```python
from build123d import *

# Parameters (mm, degrees)
SKETCH_W        = 500
SKETCH_H        = 800
PAD_DEPTH       = 850
SKETCH001_W     = 372.739898
SKETCH001_H     = 785.491455
SKETCH001_W_2   = 349.575272
SKETCH001_H_2   = 785.491421
POCKET_DEPTH    = 5
SKETCH002_W     = 52.646911
SKETCH002_H     = 789.7032
PAD001_DEPTH    = 150
SKETCH003_W     = 357.712269
SKETCH003_H     = 667.311138
POCKET001_DEPTH = 5
SKETCH004_W     = 152.212128
SKETCH004_H     = 235.528305
SKETCH004_W_2   = 136.189866
SKETCH004_H_2   = 233.926148
SKETCH004_W_3   = 157.018867
SKETCH004_H_3   = 233.926025
SKETCH004_W_4   = 136.189834
SKETCH004_H_4   = 238.732727
PAD002_DEPTH    = 10
SKETCH005_R     = 54.982504
SKETCH005_R_2   = 53.191284
SKETCH005_R_3   = 57.822478
SKETCH005_R_4   = 55.41133
PAD003_DEPTH    = 10
SKETCH006_W     = 89.111725
SKETCH006_H     = 10.483764
SKETCH006_W_2   = 87.364411
SKETCH006_H_2   = 12.231064
SKETCH006_W_3   = 94.353591
SKETCH006_H_3   = 13.978333
SKETCH006_H_4   = 10.483765
SKETCH006_W_4   = 13.978317
SKETCH006_H_5   = 96.100876
SKETCH006_W_5   = 12.230988
SKETCH006_H_6   = 94.353622
SKETCH006_H_7   = 101.342773
SKETCH006_W_6   = 10.483643
SKETCH006_H_8   = 89.111755
PAD004_DEPTH    = 10


with BuildPart() as part:
    # Sketch → Pad (new body)
    with BuildSketch(Plane.XZ):
        with Locations((250, 400)):
            Rectangle(SKETCH_W, SKETCH_H)
    extrude(amount=PAD_DEPTH)

    # Sketch001 (on Face4 of Pad) → Pocket (cut)
    with BuildSketch(Plane(origin=(0, 0, 0), x_dir=(0, 0, -1), z_dir=(-1, 0, 0))):
        with Locations((-587.422287, 426.051728)):
            Rectangle(SKETCH001_W, SKETCH001_H)
        with Locations((-205.205925, 426.051727)):
            Rectangle(SKETCH001_W_2, SKETCH001_H_2)
    extrude(amount=-POCKET_DEPTH, mode=Mode.SUBTRACT)

    # Sketch002 (on Face4 of Pocket) → Pad001 (join)
    with BuildSketch(Plane(origin=(0, 0, 0), x_dir=(1, 0, 0), z_dir=(0, 1, 0))):
        with Locations((464.799377, -400.002709)):
            Rectangle(SKETCH002_W, SKETCH002_H)
    extrude(amount=PAD001_DEPTH)

    # Sketch003 (on Face4 of Pad001) → Pocket001 (cut)
    with BuildSketch(Plane(origin=(0, 0, 0), x_dir=(1, 0, 0), z_dir=(0, 1, 0))):
        with Locations((228.396917, -394.292307)):
            Rectangle(SKETCH003_W, SKETCH003_H)
    extrude(amount=-POCKET001_DEPTH, mode=Mode.SUBTRACT)

    # Sketch004 (on Face25 of Pocket001) → Pad002 (join)
    with BuildSketch(Plane(origin=(0, -5, 0), x_dir=(1, 0, 0), z_dir=(0, 1, 0))):
        with Locations((149.261093, -246.12873)):
            Rectangle(SKETCH004_W, SKETCH004_H)
        with Locations((319.097847, -248.532074)):
            Rectangle(SKETCH004_W_2, SKETCH004_H_2)
        with Locations((148.459987, -532.12738)):
            Rectangle(SKETCH004_W_3, SKETCH004_H_3)
        with Locations((317.495598, -531.326263)):
            Rectangle(SKETCH004_W_4, SKETCH004_H_4)
    extrude(amount=PAD002_DEPTH)

    # Sketch005 (on Face43 of Pad002) → Pad003 (join)
    with BuildSketch(Plane(origin=(0, 5, 0), x_dir=(1, 0, 0), z_dir=(0, 1, 0))):
        with Locations((152.458954, -245.138535)):
            Circle(SKETCH005_R)
        with Locations((320.337128, -246.187805)):
            Circle(SKETCH005_R_2)
        with Locations((151.409729, -531.580627)):
            Circle(SKETCH005_R_3)
        with Locations((318.238647, -533.679138)):
            Circle(SKETCH005_R_4)
    extrude(amount=PAD003_DEPTH)

    # Sketch006 (on Face51 of Pad003) → Pad004 (join)
    with BuildSketch(Plane(origin=(0, 15, 0), x_dir=(1, 0, 0), z_dir=(0, 1, 0))):
        with Locations((152.860336, -247.169525)):
            Rectangle(SKETCH006_W, SKETCH006_H)
        with Locations((321.473679, -249.790474)):
            Rectangle(SKETCH006_W_2, SKETCH006_H_2)
        with Locations((157.228538, -531.977569)):
            Rectangle(SKETCH006_W_3, SKETCH006_H_3)
        with Locations((318.852737, -533.724853)):
            Rectangle(SKETCH006_W, SKETCH006_H_4)
        with Locations((158.975837, -244.548622)):
            Rectangle(SKETCH006_W_4, SKETCH006_H_5)
        with Locations((322.347336, -247.169533)):
            Rectangle(SKETCH006_W_5, SKETCH006_H_6)
        with Locations((157.228538, -533.724853)):
            Rectangle(SKETCH006_W_4, SKETCH006_H_7)
        with Locations((319.72638, -536.345795)):
            Rectangle(SKETCH006_W_6, SKETCH006_H_8)
    extrude(amount=PAD004_DEPTH)


solid = part.part
```
Can you work these out from the model? Positions are in its coordinate system, mm. A direction names the side the tool comes from. Give positions to 0.01 mm unless a question says otherwise; leave off trailing zeros. Order: outer loops, then holes, each group sorted by start corner. A loop starts at its lowest first (then second) coordinate and runs counter-clockwise, first axis right, second up. Notation, with made-up numbers: M 42,-4 L 74,-4 A22 cw 74,22 Z; hole C -1,-19.75 d1. An arc over 180 degrees is marked long. One line per item, written item: value.
1) Please list where these lines run through material, in increasing order: line 1 along X through (y, z) = (-441.5, 69.5); line 2 along Y through (x, z) = (225, 437); line 3 along Y through (x, z) = (144, 738).
Answer sheet:
line 1: x = 5 to 500
line 2: y = -850 to 5
line 3: y = -850 to 0
2) For P1, Ø8, axis at y = -299, z = 249, coming from the -X side; P2, Ø11, axis at y = 18.5, z = 513.5, coming from the -X side; P3, Ø11, axis at y = 19, z = 555.5, coming from the +X side, each with a flat end and sliding along its axis, tell me the tip position at first contact or that it passes through.
Answer sheet:
P1: stops at x = 5
P2: stops at x = 95.27
P3: stops at x = 491.12
3) I want a section at D-D, the plane z = 85.5. List the corners of the cut face in (x, y) for me, plus the area to 3 significant figures.
Answer sheet:
outline: M 0,-850 L 500,-850 L 500,0 L 491.12,0 L 491.12,150 L 438.48,150 L 438.48,0 L 407.25,0 L 407.25,-5 L 49.54,-5 L 49.54,0 L 0,0 L 0,-33.31 L 5,-33.31 L 5,-818.8 L 0,-818.8 Z
area: 427,000 mm^2
4) I want a section at A-A, the plane z = 174.5. List the corners of the cut face in (x, y) for me, plus the area to 3 significant figures.
Answer sheet:
outline: M 0,-850 L 500,-850 L 500,0 L 491.12,0 L 491.12,150 L 438.48,150 L 438.48,0 L 407.25,0 L 407.25,-5 L 387.19,-5 L 387.19,5 L 251,5 L 251,-5 L 225.37,-5 L 225.37,5 L 73.16,5 L 73.16,-5 L 49.54,-5 L 49.54,0 L 0,0 L 0,-33.31 L 5,-33.31 L 5,-818.8 L 0,-818.8 Z
area: 430,000 mm^2
5) On a 3-axis mill with a long thin cutter (end or side, diameter ignored), from which of +Z, -Z, +X, -X, +Y, -Y can I reach the whole of each face in a straight line? I mean faces 1 (the face through (5, -432, 590)), 2 (the face through (156, 25, 248)), 3 (the face through (464, 74, 5.151)), 4 (the face through (95, 5, 556)), 5 (the face through (491.123, 74, 406)). Say none if no direction works.
Answer sheet:
face 1: -X
face 2: +Z, -Z, -X, +Y
face 3: -Z, +X, -X, +Y
face 4: +Y
face 5: +Z, -Z, +X, +Y
6) I want a section at B-B, the plane y = 59.5. List the corners of the cut face in (x, z) for me, plus the area to 3 significant figures.
Answer sheet:
outline: M 438.48,5.15 L 491.12,5.15 L 491.12,794.85 L 438.48,794.85 Z
area: 41,600 mm^2
7) I want a section at C-C, the plane z = 439. List the corners of the cut face in (x, y) for me.
Answer sheet:
outline: M 0,-850 L 500,-850 L 500,0 L 491.12,0 L 491.12,150 L 438.48,150 L 438.48,0 L 407.25,0 L 407.25,-5 L 385.59,-5 L 385.59,5 L 249.4,5 L 249.4,-5 L 226.97,-5 L 226.97,5 L 69.95,5 L 69.95,-5 L 49.54,-5 L 49.54,0 L 0,0 L 0,-33.31 L 5,-33.31 L 5,-818.8 L 0,-818.8 Z
8) We'd pull the mould along Z, two halves only. Please class faces 6 (the face through (247, -419, 0)), 7 (the face through (464, 74, 794.854)), 8 (the face through (177.83, 9.93, 293.917)): released by +Z, released by -Z, zero draft, split by the parting line, or undercut.
Answer sheet:
face 6: released by -Z
face 7: released by +Z
face 8: undercut
